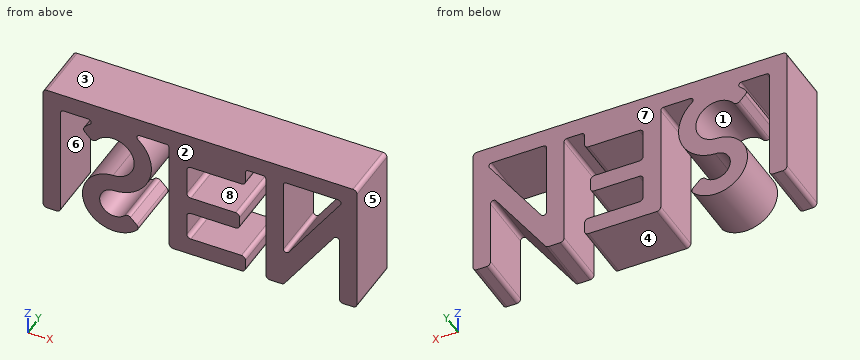
from build123d import *

# Parameters (mm, degrees)
BOSS_EXTRU_1_DEPTH = 10


with BuildPart() as part:
    # Esquisse3 → Boss.-Extru.1 (new body)
    with BuildSketch(Plane(origin=(0, 0, 0), x_dir=(1, 0, 0), z_dir=(0, 1, 0))):
        with BuildLine():
            Line((-82.4, 43.960350299), (-82.4, 24.660350299))
            Line((-82.4, 24.660350299), (-82.4, 22.360350299))
            ThreePointArc((-82.4, 22.360350299), (-82.194974747, 21.865375552), (-81.7, 21.660350299))
            Line((-81.7, 21.660350299), (-29.6, 21.660350299))
            ThreePointArc((-29.6, 21.660350299), (-29.105025253, 21.865375552), (-28.9, 22.360350299))
            Line((-28.9, 22.360350299), (-28.9, 24.660350299))
            Line((-28.9, 24.660350299), (-28.9, 43.960350299))
            ThreePointArc((-28.9, 43.960350299), (-29.105025253, 44.455325045), (-29.6, 44.660350299))
            Line((-29.6, 44.660350299), (-31.2, 44.660350299))
            ThreePointArc((-31.2, 44.660350299), (-31.694974747, 44.455325045), (-31.9, 43.960350299))
            Line((-31.9, 43.960350299), (-31.9, 32.665451753))
            ThreePointArc((-31.9, 32.665451753), (-32.234265531, 32.16295091), (-32.808648392, 32.348220639))
            Line((-32.808648392, 32.348220639), (-41.220684895, 44.361853804))
            ThreePointArc((-41.220684895, 44.361853804), (-41.470867297, 44.581257882), (-41.794091326, 44.660350299))
            Line((-41.794091326, 44.660350299), (-43.729694391, 44.660350299))
            ThreePointArc((-43.729694391, 44.660350299), (-44.224669138, 44.455325045), (-44.429694391, 43.960350299))
            Line((-44.429694391, 43.960350299), (-44.429694391, 25.160350299))
            ThreePointArc((-44.429694391, 25.160350299), (-44.576141, 24.806796908), (-44.929694391, 24.660350299))
            Line((-44.929694391, 24.660350299), (-47.4, 24.660350299))
            ThreePointArc((-47.4, 24.660350299), (-47.753553391, 24.806796908), (-47.9, 25.160350299))
            Line((-47.9, 25.160350299), (-47.9, 26.96406145))
            ThreePointArc((-47.9, 26.96406145), (-48.105025253, 27.459036196), (-48.6, 27.66406145))
            Line((-48.6, 27.66406145), (-57.2, 27.66406145))
            ThreePointArc((-57.2, 27.66406145), (-57.694974747, 27.869086703), (-57.9, 28.36406145))
            Line((-57.9, 28.36406145), (-57.9, 32.960350299))
            ThreePointArc((-57.9, 32.960350299), (-57.694974747, 33.455325045), (-57.2, 33.660350299))
            Line((-57.2, 33.660350299), (-49.6, 33.660350299))
            ThreePointArc((-49.6, 33.660350299), (-49.105025253, 33.865375552), (-48.9, 34.360350299))
            Line((-48.9, 34.360350299), (-48.9, 35.960350299))
            ThreePointArc((-48.9, 35.960350299), (-49.105025253, 36.455325045), (-49.6, 36.660350299))
            Line((-49.6, 36.660350299), (-57.2, 36.660350299))
            ThreePointArc((-57.2, 36.660350299), (-57.694974747, 36.865375552), (-57.9, 37.360350299))
            Line((-57.9, 37.360350299), (-57.9, 40.960350299))
            ThreePointArc((-57.9, 40.960350299), (-57.694974747, 41.455325045), (-57.2, 41.660350299))
            Line((-57.2, 41.660350299), (-48.6, 41.660350299))
            ThreePointArc((-48.6, 41.660350299), (-48.105025253, 41.865375552), (-47.9, 42.360350299))
            Line((-47.9, 42.360350299), (-47.9, 43.960350299))
            ThreePointArc((-47.9, 43.960350299), (-48.105025253, 44.455325045), (-48.6, 44.660350299))
            Line((-48.6, 44.660350299), (-60.2, 44.660350299))
            ThreePointArc((-60.2, 44.660350299), (-60.694974747, 44.455325045), (-60.9, 43.960350299))
            Line((-60.9, 43.960350299), (-60.9, 25.160350299))
            ThreePointArc((-60.9, 25.160350299), (-61.046446609, 24.806796908), (-61.4, 24.660350299))
            Line((-61.4, 24.660350299), (-65.9, 24.660350299))
            ThreePointArc((-65.9, 24.660350299), (-66.369202757, 24.987582324), (-66.224252839, 25.540955207))
            ThreePointArc((-66.224252839, 25.540955207), (-64.278360769, 32.64470583), (-70.174954097, 37.058316142))
            ThreePointArc((-70.174954097, 37.058316142), (-72.565676109, 40.459645131), (-68.487924516, 41.269912109))
            ThreePointArc((-68.487924516, 41.269912109), (-67.991231434, 41.058872606), (-67.492020465, 41.26388504))
            Line((-67.492020465, 41.26388504), (-66.408605494, 42.347300011))
            ThreePointArc((-66.408605494, 42.347300011), (-66.203586079, 42.839415787), (-66.404578845, 43.333189829))
            ThreePointArc((-66.404578845, 43.333189829), (-75.216844977, 41.718134484), (-70.456992958, 34.128124806))
            ThreePointArc((-70.456992958, 34.128124806), (-67.224229351, 28.944517523), (-73.29773035, 28.286390935))
            ThreePointArc((-73.29773035, 28.286390935), (-73.806166505, 28.551332862), (-74.342034946, 28.347503126))
            Line((-74.342034946, 28.347503126), (-75.273738539, 27.415799533))
            ThreePointArc((-75.273738539, 27.415799533), (-75.478062353, 26.95215404), (-75.316017422, 26.472094871))
            ThreePointArc((-75.316017422, 26.472094871), (-74.866763267, 25.988060793), (-74.369432688, 25.55357192))
            ThreePointArc((-74.369432688, 25.55357192), (-74.205711949, 24.996965493), (-74.678263963, 24.660350299))
            Line((-74.678263963, 24.660350299), (-78.9, 24.660350299))
            ThreePointArc((-78.9, 24.660350299), (-79.253553391, 24.806796908), (-79.4, 25.160350299))
            Line((-79.4, 25.160350299), (-79.4, 43.960350299))
            ThreePointArc((-79.4, 43.960350299), (-79.605025253, 44.455325045), (-80.1, 44.660350299))
            Line((-80.1, 44.660350299), (-81.7, 44.660350299))
            ThreePointArc((-81.7, 44.660350299), (-82.194974747, 44.455325045), (-82.4, 43.960350299))
        make_face()
        with BuildLine():
            Line((-41.429694391, 25.160350299), (-41.429694391, 37.760350299))
            ThreePointArc((-41.429694391, 37.760350299), (-41.08004729, 38.237208774), (-40.520118369, 38.047138517))
            Line((-40.520118369, 38.047138517), (-31.697503387, 25.447138517))
            ThreePointArc((-31.697503387, 25.447138517), (-31.663573993, 24.929475992), (-32.107079409, 24.660350299))
            Line((-32.107079409, 24.660350299), (-40.929694391, 24.660350299))
            ThreePointArc((-40.929694391, 24.660350299), (-41.283247781, 24.806796908), (-41.429694391, 25.160350299))
        make_face(mode=Mode.SUBTRACT)
    extrude(amount=BOSS_EXTRU_1_DEPTH)


solid = part.part
Input: part model. Units: mm. Frame: model coordinates. Face numbers are marked on the shaded views. A direction names the side the tool comes from. Coordinates: 2 decimals unless noted, no trailing zeros. Loops run counter-clockwise (first coordinate to the right, second up) from the corner with the lowest first, then second, coordinate; pieces in that order, holes last. Notation, with made-up numbers: (-36, -38) -> (-12, -38) arc R29 ccw to (-12, -17) -> close; hole circle Ø8 at (72, 75.25). An arc over 180 degrees is marked (long way). Write item = value, one per line. Start each with the question number.
Item 1: Cut plane D-D, the plane z = -38.75. Return loops of the section in (x, y).
Item 2: Reachability of the marked faces 4, 5, 6, 7 and 8 from +Z, -Z, +X, -X, +Y, -Y: full face, straight path, thin tool, end or side. Return the list, or none.
Item 3: Cut plane A-A, the plane x = -56. Return loops of the section in (y, z).
Item 4: Cut plane C-C, the plane x = -64.5. Return loops of the section in (y, z).
Item 5: Cut plane B-B, the plane z = -30.75. Return loops of the section in (x, y), plus the area to 3 significant figures.
Item 6: First-contact query: P1, Ø2.5, axis at x = -54.5, y = 5.5, coming from the -Z side; P2, Ø2, axis at x = -76, y = 7, coming from the -Z side; P3, Ø2.5, axis at x = -38.5, y = 3.5, coming from the -Z side. Flat tips, straight axial feed; report the tip coordinate or a pass-through.
Item 7: Mould query, pull axis Z, two halves, no side actions, for the marked faces 1, 2 and 3. Classes: pulls with the +Z half, pulls with the -Z half, needs draft (parallel to the pull), parting line crosses it, or undercut.
Item 8: Material intervals for line 1 (Z direction, x = -70.5, y = 6.75); line 2 (Z direction, x = -51, y = 2); line 3 (X direction, y = 1.5, z = -42.5), sorted ascending.
Ans:
q1.outline = (-82.4, 0) -> (-79.4, 0) -> (-79.4, 10) -> (-82.4, 10) -> close; (-75.62, 0) -> (-72.62, 0) -> (-72.62, 10) -> (-75.62, 10) -> close; (-60.9, 0) -> (-57.9, 0) -> (-57.9, 10) -> (-60.9, 10) -> close; (-44.43, 0) -> (-37.29, 0) -> (-37.29, 10) -> (-44.43, 10) -> close; (-31.9, 0) -> (-28.9, 0) -> (-28.9, 10) -> (-31.9, 10) -> close
q2.face_4 = -Z, +X, +Y, -Y
q2.face_5 = +Z, -Z, +X, +Y, -Y
q2.face_6 = -Z, +Y, -Y
q2.face_7 = +Z, -Z, +X, -X, +Y
q2.face_8 = +Y, -Y
q3.outline = (0, -44.66) -> (10, -44.66) -> (10, -41.66) -> (0, -41.66) -> close; (0, -36.66) -> (10, -36.66) -> (10, -33.66) -> (0, -33.66) -> close; (0, -27.66) -> (10, -27.66) -> (10, -21.66) -> (0, -21.66) -> close
q4.outline = (0, -33.21) -> (10, -33.21) -> (10, -27.84) -> (0, -27.84) -> close; (0, -24.66) -> (10, -24.66) -> (10, -21.66) -> (0, -21.66) -> close
q5.outline = (-82.4, 0) -> (-79.4, 0) -> (-79.4, 10) -> (-82.4, 10) -> close; (-66.87, 0) -> (-63.93, 0) -> (-63.93, 10) -> (-66.87, 10) -> close; (-60.9, 0) -> (-57.9, 0) -> (-57.9, 10) -> (-60.9, 10) -> close; (-44.43, 0) -> (-41.43, 0) -> (-41.43, 10) -> (-44.43, 10) -> close; (-35.41, 0) -> (-28.9, 0) -> (-28.9, 10) -> (-35.41, 10) -> close
q5.area = 185 mm²
q6.P1 = -44.66
q6.P2 = -42.16
q6.P3 = -42.26
q7.face_1 = undercut
q7.face_2 = needs draft
q7.face_3 = pulls with the +Z half
q8.line_1 = -44.94 to -42.01, -37.07 to -34.13, -26.92 to -21.66
q8.line_2 = -44.66 to -41.66, -36.66 to -33.66, -27.66 to -21.66
q8.line_3 = -82.4 to -79.4, -74.79 to -66.29, -60.9 to -47.9, -44.43 to -39.92, -31.9 to -28.9
